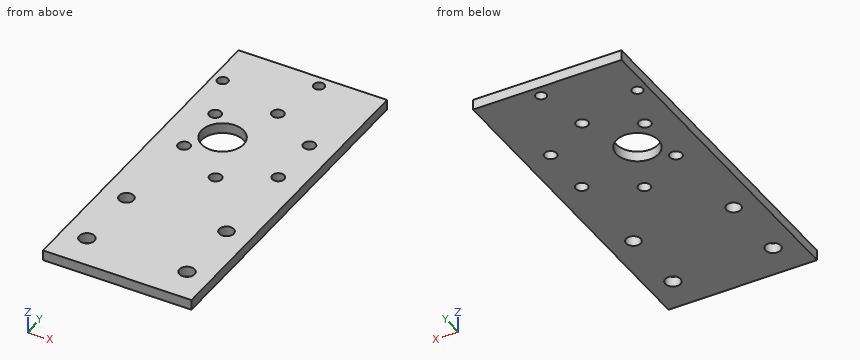
from build123d import *

# Parameters (mm, degrees)
SKETCH_1_W          = 40
SKETCH_1_H          = 29
EXTRUDE_1_DEPTH     = 3
CUT_EXTRUDE_1_DEPTH = 3
SKETCH_3_W          = 40
SKETCH_3_H          = 3
EXTRUDE_2_DEPTH     = 10
SKETCH_4_W          = 40
SKETCH_4_H          = 3
EXTRUDE_3_DEPTH     = 10
SKETCH_6_W          = 3
SKETCH_6_H          = 49
EXTRUDE_5_DEPTH     = 42
SKETCH_8_W          = 3
SKETCH_8_H          = 49
EXTRUDE_6_DEPTH     = 2
SKETCH_9_W          = 3
SKETCH_9_H          = 49
EXTRUDE_7_DEPTH     = 2
SKETCH_10_W         = 86
SKETCH_10_H         = 3
EXTRUDE_8_DEPTH     = 10
SKETCH_11_W         = 86
SKETCH_11_H         = 3
EXTRUDE_9_DEPTH     = 10
SKETCH_7_R          = 1.75
SKETCH_7_R_2        = 6.1
CUT_EXTRUDE_4_DEPTH = 10
SKETCH_14_W         = 3
SKETCH_14_H         = 69
CUT_EXTRUDE_5_DEPTH = 43
SKETCH_17_W         = 43
SKETCH_17_H         = 3
EXTRUDE_10_DEPTH    = 20
SKETCH_18_R         = 2.1
CUT_EXTRUDE_6_DEPTH = 10
SKETCH_20_W         = 43
SKETCH_20_H         = 3
EXTRUDE_11_DEPTH    = 10
SKETCH_21_W         = 43
SKETCH_21_H         = 3
CUT_EXTRUDE_7_DEPTH = 10
SKETCH_22_R         = 2.2
CUT_EXTRUDE_8_DEPTH = 10
SKETCH_24_W         = 43
SKETCH_24_H         = 3
EXTRUDE_12_DEPTH    = 10
SKETCH_25_R         = 1.55
CUT_EXTRUDE_9_DEPTH = 10


with BuildPart() as part:
    # ｽｹｯﾁ1 → ﾎﾞｽ - 押し出し1 (new body)
    with BuildSketch(Plane.XY):
        Rectangle(SKETCH_1_W, SKETCH_1_H)
    extrude(amount=EXTRUDE_1_DEPTH)

    # ｽｹｯﾁ2 → ｶｯﾄ - 押し出し1 (cut)
    with BuildSketch(Plane.XY.offset(3)):
        with BuildLine():
            ThreePointArc((-14.4, 10.5), (-15.01507576, 11.98492424), (-16.5, 12.6))
            Line((-16.5, 12.6), (-16.5, 10.5))
            Line((-16.5, 10.5), (-18.6, 10.5))
            ThreePointArc((-18.6, 10.5), (-16.5, 8.4), (-14.4, 10.5))
        make_face()
        with BuildLine():
            Line((-16.5, 10.5), (-16.5, 12.6))
            ThreePointArc((-16.5, 12.6), (-17.98492424, 11.98492424), (-18.6, 10.5))
            Line((-18.6, 10.5), (-16.5, 10.5))
        make_face()
        with BuildLine():
            ThreePointArc((-18.6, -10.5), (-17.98492424, -11.98492424), (-16.5, -12.6))
            Line((-16.5, -12.6), (-16.5, -10.5))
            Line((-16.5, -10.5), (-18.6, -10.5))
        make_face()
        with BuildLine():
            Line((-16.5, -10.5), (-16.5, -12.6))
            ThreePointArc((-16.5, -12.6), (-15.01507576, -11.98492424), (-14.4, -10.5))
            ThreePointArc((-14.4, -10.5), (-16.5, -8.4), (-18.6, -10.5))
            Line((-18.6, -10.5), (-16.5, -10.5))
        make_face()
        with BuildLine():
            ThreePointArc((18.6, -10.5), (15.01507576, -9.01507576), (16.5, -12.6))
            Line((16.5, -12.6), (16.5, -10.5))
            Line((16.5, -10.5), (18.6, -10.5))
        make_face()
        with BuildLine():
            Line((16.5, -10.5), (16.5, -12.6))
            ThreePointArc((16.5, -12.6), (17.98492424, -11.98492424), (18.6, -10.5))
            Line((18.6, -10.5), (16.5, -10.5))
        make_face()
        with BuildLine():
            ThreePointArc((18.6, 10.5), (17.98492424, 11.98492424), (16.5, 12.6))
            Line((16.5, 12.6), (16.5, 10.5))
            Line((16.5, 10.5), (18.6, 10.5))
        make_face()
        with BuildLine():
            Line((16.5, 10.5), (16.5, 12.6))
            ThreePointArc((16.5, 12.6), (15.01507576, 9.01507576), (18.6, 10.5))
            Line((18.6, 10.5), (16.5, 10.5))
        make_face()
    extrude(amount=-CUT_EXTRUDE_1_DEPTH, mode=Mode.SUBTRACT)

    # ｽｹｯﾁ3 → ﾎﾞｽ - 押し出し2 (add)
    with BuildSketch(Plane.XZ.offset(14.5)):
        with Locations((0, 1.5)):
            Rectangle(SKETCH_3_W, SKETCH_3_H)
    extrude(amount=EXTRUDE_2_DEPTH)

    # ｽｹｯﾁ4 → ﾎﾞｽ - 押し出し3 (add)
    with BuildSketch(Plane(origin=(0, 14.5, 0), x_dir=(1, 0, 0), z_dir=(0, 1, 0))):
        with Locations((0, -1.5)):
            Rectangle(SKETCH_4_W, SKETCH_4_H)
    extrude(amount=EXTRUDE_3_DEPTH)

    # ｽｹｯﾁ6 → ﾎﾞｽ - 押し出し5 (add)
    with BuildSketch(Plane(origin=(20, 0, 0), x_dir=(0, 0, -1), z_dir=(1, 0, 0))):
        with Locations((-1.5, 0)):
            Rectangle(SKETCH_6_W, SKETCH_6_H)
    extrude(amount=EXTRUDE_5_DEPTH)

    # ｽｹｯﾁ8 → ﾎﾞｽ - 押し出し6 (add)
    with BuildSketch(Plane.ZY.offset(20)):
        with Locations((1.5, 0)):
            Rectangle(SKETCH_8_W, SKETCH_8_H)
    extrude(amount=EXTRUDE_6_DEPTH)

    # ｽｹｯﾁ9 → ﾎﾞｽ - 押し出し7 (add)
    with BuildSketch(Plane(origin=(62, 0, 0), x_dir=(0, 0, -1), z_dir=(1, 0, 0))):
        with Locations((-1.5, 0)):
            Rectangle(SKETCH_9_W, SKETCH_9_H)
    extrude(amount=EXTRUDE_7_DEPTH)

    # ｽｹｯﾁ10 → ﾎﾞｽ - 押し出し8 (add)
    with BuildSketch(Plane.XZ.offset(24.5)):
        with Locations((21, 1.5)):
            Rectangle(SKETCH_10_W, SKETCH_10_H)
    extrude(amount=EXTRUDE_8_DEPTH)

    # ｽｹｯﾁ11 → ﾎﾞｽ - 押し出し9 (add)
    with BuildSketch(Plane(origin=(0, 24.5, 0), x_dir=(1, 0, 0), z_dir=(0, 1, 0))):
        with Locations((21, -1.5)):
            Rectangle(SKETCH_11_W, SKETCH_11_H)
    extrude(amount=EXTRUDE_9_DEPTH)

    # ｽｹｯﾁ7 → ｶｯﾄ - 押し出し4 (cut)
    with BuildSketch(Plane.XY.offset(3)):
        with Locations((56.745697969, 7.875)):
            Circle(SKETCH_7_R)
        with Locations((56.745697969, -7.875)):
            Circle(SKETCH_7_R)
        with Locations((36.10579786, 0)):
            Circle(SKETCH_7_R_2)
        with Locations((43.10579786, 15.75)):
            Circle(SKETCH_7_R)
        with Locations((43.10579786, -15.75)):
            Circle(SKETCH_7_R)
        with Locations((29.46589775, 7.875)):
            Circle(SKETCH_7_R)
        with Locations((29.46589775, -7.875)):
            Circle(SKETCH_7_R)
    extrude(amount=-CUT_EXTRUDE_4_DEPTH, mode=Mode.SUBTRACT)

    # ｽｹｯﾁ14 → ｶｯﾄ - 押し出し5 (cut)
    with BuildSketch(Plane.ZY.offset(22)):
        with Locations((1.5, 0)):
            Rectangle(SKETCH_14_W, SKETCH_14_H)
    extrude(amount=-CUT_EXTRUDE_5_DEPTH, mode=Mode.SUBTRACT)

    # ｽｹｯﾁ17 → ﾎﾞｽ - 押し出し10 (add)
    with BuildSketch(Plane.XZ.offset(34.5)):
        with Locations((42.5, 1.5)):
            Rectangle(SKETCH_17_W, SKETCH_17_H)
    extrude(amount=EXTRUDE_10_DEPTH)

    # ｽｹｯﾁ18 → ｶｯﾄ - 押し出し6 (cut)
    with BuildSketch(Plane.XY.offset(3)):
        with Locations((28, -34.5)):
            Circle(SKETCH_18_R)
        with Locations((57, -34.5)):
            Circle(SKETCH_18_R)
    extrude(amount=-CUT_EXTRUDE_6_DEPTH, mode=Mode.SUBTRACT)

    # ｽｹｯﾁ20 → ﾎﾞｽ - 押し出し11 (add)
    with BuildSketch(Plane.XZ.offset(54.5)):
        with Locations((42.5, 1.5)):
            Rectangle(SKETCH_20_W, SKETCH_20_H)
    extrude(amount=EXTRUDE_11_DEPTH)

    # ｽｹｯﾁ21 → ｶｯﾄ - 押し出し7 (cut)
    with BuildSketch(Plane(origin=(0, 34.5, 0), x_dir=(1, 0, 0), z_dir=(0, 1, 0))):
        with Locations((42.5, -1.5)):
            Rectangle(SKETCH_21_W, SKETCH_21_H)
    extrude(amount=-CUT_EXTRUDE_7_DEPTH, mode=Mode.SUBTRACT)

    # ｽｹｯﾁ22 → ｶｯﾄ - 押し出し8 (cut)
    with BuildSketch(Plane.XY.offset(3)):
        with Locations((28, -54.5)):
            Circle(SKETCH_22_R)
        with Locations((57, -54.5)):
            Circle(SKETCH_22_R)
    extrude(amount=-CUT_EXTRUDE_8_DEPTH, mode=Mode.SUBTRACT)

    # ｽｹｯﾁ24 → ﾎﾞｽ - 押し出し12 (add)
    with BuildSketch(Plane(origin=(0, 24.5, 0), x_dir=(1, 0, 0), z_dir=(0, 1, 0))):
        with Locations((42.5, -1.5)):
            Rectangle(SKETCH_24_W, SKETCH_24_H)
    extrude(amount=EXTRUDE_12_DEPTH)

    # ｽｹｯﾁ25 → ｶｯﾄ - 押し出し9 (cut)
    with BuildSketch(Plane.XY.offset(3)):
        with Locations((24, 21.2)):
            Circle(SKETCH_25_R)
        with Locations((46.2, 31.2)):
            Circle(SKETCH_25_R)
    extrude(amount=-CUT_EXTRUDE_9_DEPTH, mode=Mode.SUBTRACT)


solid = part.part
Geometry: final body of the model. Coordinates: model frame, mm. Give positions to 0.01 mm unless a question says otherwise; leave off trailing zeros. Write each loop counter-clockwise with the first axis right and the second up, starting at its lowest first coordinate (ties: lowest second). Pieces come first, ordered by that corner, then holes.
(1) Cut plane B-B, the plane x = 46.2. Return loops of the section in (y, z), then the cut area to 3 significant figures.
(2) Cut plane A-A, the plane y = -15.75. Return loops of the section in (x, z), then the cut area to 4 significant figures.
(3) Ray query, line 1 (X direction, y = 8, z = 1.5); line 2 (Y direction, x = 46.2, z = 1.1); line 3 (Y direction, x = 57.5, z = 0.4). Return the intervals inside material, ascending.
(4) Cut plane C-C, the plane z = 2.5. Give the number of separate pieces and of enclosed holes in the cut face, then the cut area to 3 significant figures.
Values follow:
1. outline: (-64.5, 0) - (29.65, 0) - (29.65, 3) - (-64.5, 3) - close; (32.75, 0) - (34.5, 0) - (34.5, 3) - (32.75, 3) - close
1. area: 288 mm2
2. outline: (21, 0) - (41.36, 0) - (41.36, 3) - (21, 3) - close; (44.86, 0) - (64, 0) - (64, 3) - (44.86, 3) - close
2. area: 118.5 mm2
3. line 1: x = 21 to 27.72, 31.21 to 55, 58.49 to 64
3. line 2: y = -64.5 to 29.65, 32.75 to 34.5
3. line 3: y = -64.5 to -56.64, -52.36 to -36.54, -32.46 to -9.45, -6.3 to 6.3, 9.45 to 34.5
4. separate pieces: 1
4. enclosed holes: 13
4. area: 4,010 mm2
